```python
from build123d import *

# Parameters (mm, degrees)
F0_R      = 47.625
F1_DEPTH  = 6.35
F3_DEPTH  = 4.2545
F5_W      = 19.05
F5_H      = 6.35
F6_DEPTH  = 6.35
F8_DEPTH  = 19.05
F9_R      = 3.175
F10_DEPTH = 19.05
F4_R      = 1.5875
F11_DEPTH = 25.4


with BuildPart() as f1:
    # F0 (on Top) → F1 (new body)
    with BuildSketch(Plane.XY):
        Circle(F0_R)
    extrude(amount=F1_DEPTH)

    # F2 (on face) → F3 (cut)
    with BuildSketch(Plane.XY.offset(6.35)):
        with BuildLine():
            ThreePointArc((12.7, 45.900442536), (0, 47.625), (-12.7, 45.900442536))
            Line((-12.7, 45.900442536), (-12.7, 12.7))
            Line((-12.7, 12.7), (-45.900442536, 12.7))
            ThreePointArc((-45.900442536, 12.7), (-47.625, 0), (-45.900442536, -12.7))
            Line((-45.900442536, -12.7), (-12.7, -12.7))
            Line((-12.7, -12.7), (-12.7, -45.900442536))
            ThreePointArc((-12.7, -45.900442536), (0, -47.625), (12.7, -45.900442536))
            Line((12.7, -45.900442536), (12.7, -12.7))
            Line((12.7, -12.7), (45.900442536, -12.7))
            ThreePointArc((45.900442536, -12.7), (47.1918912567, -6.4082778195), (47.625, 0))
            ThreePointArc((47.625, 0), (47.1918912567, 6.4082778195), (45.900442536, 12.7))
            Line((45.900442536, 12.7), (12.7, 12.7))
            Line((12.7, 12.7), (12.7, 45.900442536))
        make_face()
    extrude(amount=-F3_DEPTH, mode=Mode.SUBTRACT)

    # F5 (on face) → F6 (join)
    with BuildSketch(Plane(origin=(0, 0, 0), x_dir=(1, 0, 0), z_dir=(0, 0, -1))):
        with Locations((0, 0.1347091747)):
            Rectangle(F5_W, F5_H)
    extrude(amount=F6_DEPTH)

    # F7 (on face) → F8 (join)
    with BuildSketch(Plane(origin=(-9.525, 0, 0), x_dir=(0, -1, 0), z_dir=(-1, 0, 0))):
        with BuildLine():
            ThreePointArc((-3.0402908253, -1.0568323894), (-3.2416549215, -12.0919341109), (6.35, -6.6316984594))
            ThreePointArc((6.35, -6.6316984594), (5.5380119745, -3.5247830485), (3.3097091747, -1.2124434203))
            Line((3.3097091747, -1.2124434203), (3.3097091747, -6.35))
            Line((3.3097091747, -6.35), (-3.0402908253, -6.35))
            Line((-3.0402908253, -6.35), (-3.0402908253, -1.0568323894))
        make_face()
    extrude(amount=-F8_DEPTH)

    # F9 (on face) → F10 (cut)
    with BuildSketch(Plane.YZ.offset(9.525)):
        with Locations((0, -6.6316984594)):
            Circle(F9_R)
    extrude(amount=-F10_DEPTH, mode=Mode.SUBTRACT)

    # F4 (on face) → F11 (cut)
    with BuildSketch(Plane.XY.offset(2.0955)):
        with Locations((-38.1, 0)):
            Circle(F4_R)
        with Locations((-25.4, 0)):
            Circle(F4_R)
        with Locations((0, -25.4)):
            Circle(F4_R)
        with Locations((0, -38.1)):
            Circle(F4_R)
        with Locations((25.4, 0)):
            Circle(F4_R)
        with Locations((38.1, 0)):
            Circle(F4_R)
        with Locations((0, 25.4)):
            Circle(F4_R)
        with Locations((0, 38.1)):
            Circle(F4_R)
    extrude(amount=-F11_DEPTH, mode=Mode.SUBTRACT)


solid = f1.part
```
Design review of the part built by this model. Coordinates are the model's own, in mm. A direction names the side the tool comes from. Give positions to 0.01 mm unless a question says otherwise; leave off trailing zeros. Loops run counter-clockwise (first coordinate to the right, second up) from the corner with the lowest first, then second, coordinate; pieces in that order, holes last. Notation, with made-up numbers: M 86.25,47 L 138.25,47 A26 ccw 138.25,86 Z; hole C 51.25,9.5 d9. An arc over 180 degrees is marked long. Return JSON: item names as keys, results as strings. Group by question number.
Item 1: We need section A-A (x = 0). Give the number of separate pieces and of enclosed holes in the cut face, and give its area (3 significant figures).
Item 2: We need section C-C (z = -8.5). Give the boundary of the cut face in (x, y) (3 decimals), and give its area (3 significant figures).
Item 3: Mouldability with a two-part tool opening along Y and no side actions: class faces 1 (the flat face through (-26, -25, 6.35)), 2 (the cylindrical face through (-0.207, 26.974, 1.062)), 3 (the cylindrical face through (45.426, 14.305, 3.131)) as released by +Y, released by -Y, zero draft, split by the parting line, or undercut.
Item 4: Insertion check: pin 1 Ø3.5 at (x, y) = (0, 38.1) entering from -Z; pin 2 Ø10 at (x, z) = (-24, 2) entering from -Y; pin 3 Ø3 at (x, z) = (-36.5, 4) entering from -Y; pin 4 Ø4 at (y, z) = (0, -6.63) entering from +X. Each pin has a flat end and moves straight along its axis. Give the tip position at first contact, or say it passes through.
Item 5: Tool access review of faces 4 (the flat face through (-29, 12.7, 4)), 5 (the flat face through (25, -25, 6.35)), 6 (the flat face through (12.7, 29, 4)), 7 (the flat face through (9.525, 3, -5)): name each direction out of +Z, -Z, +X, -X, +Y, -Y from which nothing blocks a thin tool from reaching the whole face with its end or side.
Item 6: For probe 1 along Y at (x, z) = (0, 0.7) (1 decimal); probe 2 along Z at (x, y) = (-13, 37); probe 3 along Y at (x, z) = (41, 3.5), list the stretches that pass through material, from the lowest coordinate up.
Item 7: We need section B-B (y = 0). Give the boundary of the cut face in (x, z) (1 decimal).
Output:
{
 "1": {"separate pieces": "5", "enclosed holes": "1", "area": "272 mm^2"},
 "2": {"outline": "M -9.525,-6.069 L 9.525,-6.069 L 9.525,-2.567 L -9.525,-2.567 Z; M -9.525,2.567 L 9.525,2.567 L 9.525,6.069 L -9.525,6.069 Z", "area": "133 mm^2"},
 "3": {"face 1": "zero draft", "face 2": "undercut", "face 3": "split by the parting line"},
 "4": {"pin 1": "stops at z = 0", "pin 2": "stops at y = -43.67", "pin 3": "stops at y = -32.3", "pin 4": "passes through"},
 "5": {"face 4": "+Z, +X, -X", "face 5": "+Z, +X, -X, +Y, -Y", "face 6": "+Z, +Y, -Y", "face 7": "-Z, +X, +Y, -Y"},
 "6": {"probe 1": "y = -47.6 to -39.7, -36.5 to -27, -23.8 to 23.8, 27 to 36.5, 39.7 to 47.6", "probe 2": "z = 0 to 6.35", "probe 3": "y = -24.23 to -12.7, 12.7 to 24.23"},
 "7": {"outline": "M -47.6,0 L -39.7,0 L -39.7,2.1 L -47.6,2.1 Z; M -36.5,0 L -27,0 L -27,2.1 L -36.5,2.1 Z; M -23.8,0 L -9.5,0 L -9.5,-3.5 L 9.5,-3.5 L 9.5,0 L 23.8,0 L 23.8,2.1 L -23.8,2.1 Z; M -9.5,-13 L 9.5,-13 L 9.5,-9.8 L -9.5,-9.8 Z; M 27,0 L 36.5,0 L 36.5,2.1 L 27,2.1 Z; M 39.7,0 L 47.6,0 L 47.6,2.1 L 39.7,2.1 Z"}
}
